CAD build for the part. Positions are in the model's coordinates, mm. Give positions to 0.01 mm unless a question says otherwise; leave off trailing zeros. Order: outer loops, then holes, each group sorted by start corner. A loop starts at its lowest first (then second) coordinate and runs counter-clockwise, first axis right, second up.
Item 1: Band-saw the part on A-A on y = -194.5. Give the cut face in (x, z), plus the area to 3 significant figures.
Item 2: Flat gauge pins, fed straight in: P1, Ø2, axis at y = 20.5, z = 32.5, coming from the -X side; P2, Ø6, axis at x = 25.5, z = 50.5, coming from the +Y side; P3, Ø10, axis at x = 24.5, z = -12.5, coming from the -Y side. Where does each tip first touch, or does it go through?
Item 3: Wall check: L1, parallel to Y at x = -50, z = 46; L2, parallel to Y at x = -63.5, z = -7.5; L3, parallel to Z at x = -26, y = 53. Give the ranges that are in metal, low to high.
```python
from build123d import *

# Parameters (mm, degrees)
F0_R      = 74.741234
F1_DEPTH  = 76.2
F2_R      = 73.515954
F1_FACE_R = 1.22528
F3_DEPTH  = 247.674868


with BuildPart() as f1:
    # F0 (on Front) → F1 (new body, symmetric)
    with BuildSketch(Plane.XZ):
        Circle(F0_R)
    extrude(amount=F1_DEPTH, both=True)

    # F2
    f2_edges = [f1.edges().sort_by_distance(p)[0] for p in [
        (-74.741234, 76.2, 0),
        (74.741234, 0, 0),
        (-74.741234, -76.2, 0),
    ]]
    fillet(f2_edges, radius=F2_R)

    # F1_face (on face) → F3 (join)
    with BuildSketch(Plane.XZ.offset(76.2)):
        Circle(F1_FACE_R)
    extrude(amount=F3_DEPTH)


solid = f1.part
```
The answers:
1. outline: circle Ø2.45 at (0, 0)
1. area: 4.72 mm2
2. P1: stops at x = -65.43
2. P2: stops at y = 54.3
2. P3: stops at y = -73.05
3. L1: y = -33.56 to 33.56
3. L2: y = -41.04 to 41.04
3. L3: z = -48.27 to 48.27
